Design review of the part built by this model. Coordinates are the model's own, in mm. A direction names the side the tool comes from. Give positions to 0.01 mm unless a question says otherwise; leave off trailing zeros. Write each loop counter-clockwise with the first axis right and the second up, starting at its lowest first coordinate (ties: lowest second). Pieces come first, ordered by that corner, then holes. Notation, with made-up numbers: M 88.5,24 L 101.5,24 A14 cw 101.5,31 Z; hole C -39.75,3 d11. An arc over 180 degrees is marked long. Write each question's results on one line, items separated by ' | '. Start each with the question number.
from build123d import *


with BuildPart() as part:
    # Sketch1 → Revolve1 (revolve)
    with BuildSketch(Plane.XY):
        Polygon((-29.804083682, 0), (-29.804083682, 1.534627615), (-28.915615063, 1.534627615), (-28.915615063, 2.665405858), (-27.623297071, 2.665405858), (-27.623297071, 4.765422594), (-26.694443515, 5.694276151), (-24.647883682, 5.694276151), (-24.647883682, 17.907), (-7.071083682, 17.907), (-7.071083682, 18.669), (19.979916318, 18.669), (19.979916318, 17.907), (25.440916318, 17.907), (25.440916318, 6.477), (29.809716318, 6.477), (29.809716318, 1.5875), (38.140916318, 1.5875), (38.140916318, 0), align=None)
    revolve(axis=Axis((-37.638761506, 0, 0), (1, 0, 0)))


solid = part.part
Q1. For faces 1 (the flat face through (38.141, 0, 0)), 2 (the cylindrical face through (-15.74, -3.88, -17.48)), 3 (the cylindrical face through (22.75, -3.88, -17.48)), list the 3-axis set-ups (+Z, -Z, +X, -X, +Y, -Y) from which the entire face can be reached by the end or side of a thin tool; tool diameter is ignored.
Q2. We need section C-C on x = -21.5. Write out the cut boundary in (y, z).
Q3. We need section D-D on y = -10. Write out the cut boundary in (x, z), and give its area (3 significant figures).
Q4. For pin 1 Ø6 at (x, z) = (-9.5, -7) entering from -Y; pin 2 Ø10 at (y, z) = (7, -4.5) entering from +X; pin 3 Ø6 at (y, z) = (11.5, -12.5) entering from +X, all flat-tipped, find the tip position at first contact; note any pin that passes through.
Q5. Wall thickness on line 1 along X through (y, z) = (-8.5, 8.5); line 2 along Z through (x, y) = (28, -4.5); line 3 along Y through (x, z) = (-6.5, -4.5): over which ranges is each line inside the solid? List them lowest first. Write a range as from..to.
Answer sheet:
1) face 1: +Z, -Z, +X, +Y, -Y | face 2: -X | face 3: +X
2) outline: C 0,0 d35.81
3) outline: M -24.65,-14.85 L -7.07,-14.85 L -7.07,-15.76 L 19.98,-15.76 L 19.98,-14.85 L 25.44,-14.85 L 25.44,14.85 L 19.98,14.85 L 19.98,15.76 L -7.07,15.76 L -7.07,14.85 L -24.65,14.85 Z | area: 1,540 mm^2
4) pin 1: y = -17.92 | pin 2: x = 29.81 | pin 3: x = 25.44
5) line 1: -24.65..25.44 | line 2: -4.66..4.66 | line 3: -18.12..18.12
